```python
from build123d import *

# Parameters (mm, degrees)
BOSS_EXTRUDE1_DEPTH      = 4.5
BOSS_EXTRUDE1_DEPTH_BACK = 4.5
SKETCH3_R                = 1.75
CUT_EXTRUDE1_DEPTH       = 4
FILLET1_R                = 2
SKETCH4_R                = 8.25
CUT_EXTRUDE2_DEPTH       = 2.7
CUT_EXTRUDE2_DEPTH_BACK  = 2.7


with BuildPart() as part:
    # Sketch2 → Boss-Extrude1 (new body, two sides)
    with BuildSketch(Plane(origin=(0, 0, 0), x_dir=(0, 0, -1), z_dir=(1, 0, 0))) as boss_extrude1_sk:
        with BuildLine():
            Line((9.539392014, 1.5), (15.5, 1.5))
            Line((15.5, 1.5), (15.5, -1.5))
            Line((15.5, -1.5), (7, -1.5))
            ThreePointArc((7, -1.5), (0, 5.5), (-7, -1.5))
            Line((-7, -1.5), (-15.5, -1.5))
            Line((-15.5, -1.5), (-15.5, 1.5))
            Line((-15.5, 1.5), (-9.539392014, 1.5))
            ThreePointArc((-9.539392014, 1.5), (0, 8.5), (9.539392014, 1.5))
        make_face()
    extrude(amount=BOSS_EXTRUDE1_DEPTH)
    extrude(boss_extrude1_sk.sketch, amount=-BOSS_EXTRUDE1_DEPTH_BACK)

    # Sketch3 → Cut-Extrude1 (cut, through all)
    with BuildSketch(Plane(origin=(0, 1.5, 0), x_dir=(1, 0, 0), z_dir=(0, 1, 0))):
        with Locations((0, 12.5)):
            Circle(SKETCH3_R)
        with Locations((0, -12.5)):
            Circle(SKETCH3_R)
    extrude(amount=-CUT_EXTRUDE1_DEPTH, mode=Mode.SUBTRACT)

    # Fillet1
    fillet1_edges = [part.edges().sort_by_distance(p)[0] for p in [
        (4.5, 0, -15.5),
        (-4.5, 0, 15.5),
        (4.5, 0, 15.5),
        (-4.5, 0, -15.5),
    ]]
    fillet(fillet1_edges, radius=FILLET1_R)

    # Sketch4 → Cut-Extrude2 (cut, two sides)
    with BuildSketch(Plane(origin=(0, 0, 0), x_dir=(0, 0, -1), z_dir=(1, 0, 0))) as cut_extrude2_sk:
        with Locations((0, -1.5)):
            Circle(SKETCH4_R)
    extrude(amount=CUT_EXTRUDE2_DEPTH, mode=Mode.SUBTRACT)
    extrude(cut_extrude2_sk.sketch, amount=-CUT_EXTRUDE2_DEPTH_BACK, mode=Mode.SUBTRACT)


solid = part.part
```
The model under review builds one solid part; all positions refer to its coordinate system, in mm. A direction names the side the tool comes from. Round coordinates to 2 decimals unless told otherwise and drop trailing zeros. Loops run counter-clockwise (first coordinate to the right, second up) from the corner with the lowest first, then second, coordinate; pieces in that order, holes last. Notation, with made-up numbers: (-27.75, -36.5) -> (21.25, -36.5) arc R24 ccw to (21.25, -16.5) -> close; hole circle Ø3 at (20.25, -29). An arc over 180 degrees is marked (long way). Answer as a JSON object with one key per item and string values. Group by question number.
1) For line 1 (X direction, y = 0.6, z = -12.5); line 2 (Z direction, x = 0, y = -0.65); line 3 (X direction, y = 4, z = -5.5), list the stretches that pass through material, from the lowest coordinate up. Write a range as [from, to].
2) We need section B-B on z = 0. Write out the cut boundary in (x, y), then the cut area to 4 significant figures.
3) We need section D-D on y = 3.75. Write out the cut boundary in (x, z), then the cut area to 3 significant figures.
4) For pin 1 Ø1 at (y, z) = (6.5, -7) entering from -X; pin 2 Ø1.8 at (x, z) = (1.5, -12) entering from +Y, all flat-tipped, find the tip position at first contact; note any pin that passes through.
5) We need section C-C on y = 0. Write out the cut boundary in (x, z).
6) We need section A-A on z = -12.5. Write out the cut boundary in (x, y), then the cut area to 3 significant figures.
7) For faces 1 (the face through (3.93, -0.02, -14.9)), 2 (the face through (0.1, 1.5, 10.6)), 3 (the face through (0, 1.5, -10)), 4 (the face through (-3.93, -0.02, -14.9)), 5 (the face through (2.7, 6, 0)), list the 3-axis set-ups (+Z, -Z, +X, -X, +Y, -Y) from which the entire face can be reached by the end or side of a thin tool; tool diameter is ignored.
8) Mouldability with a two-part tool opening along Z and no side actions: class faces 6 (the face through (-2.7, 6, 0)), 7 (the face through (-4.5, 6, 0)), 8 (the face through (-3.93, 0.02, 14.9)), 9 (the face through (3.61, 5.5, -0.15)) as released by +Z, released by -Z, zero draft, split by the parting line, or undercut.
Result set:
{
 "1": {"line 1": "[-4.5, -1.75], [1.75, 4.5]", "line 2": "[-15.5, -14.25], [-10.75, -8.21], [8.21, 10.75], [14.25, 15.5]", "line 3": "[-4.5, -2.7], [2.7, 4.5]"},
 "2": {"outline": "(-4.5, 5.5) -> (-2.7, 5.5) -> (-2.7, 6.75) -> (2.7, 6.75) -> (2.7, 5.5) -> (4.5, 5.5) -> (4.5, 8.5) -> (-4.5, 8.5) -> close", "area": "20.25 mm²"},
 "3": {"outline": "(-4.5, -8.51) -> (4.5, -8.51) -> (4.5, -4.63) -> (2.7, -4.63) -> (2.7, -6.36) -> (-2.7, -6.36) -> (-2.7, -4.63) -> (-4.5, -4.63) -> close; (-4.5, 4.63) -> (-2.7, 4.63) -> (-2.7, 6.36) -> (2.7, 6.36) -> (2.7, 4.63) -> (4.5, 4.63) -> (4.5, 8.51) -> (-4.5, 8.51) -> close", "area": "51.1 mm²"},
 "4": {"pin 1": "through", "pin 2": "y = 1.5"},
 "5": {"outline": "(-4.5, -13.5) arc R2 ccw to (-2.5, -15.5) -> (2.5, -15.5) arc R2 ccw to (4.5, -13.5) -> (4.5, -6.84) -> (2.7, -6.84) -> (2.7, -8.11) -> (-2.7, -8.11) -> (-2.7, -6.84) -> (-4.5, -6.84) -> close; (-4.5, 6.84) -> (-2.7, 6.84) -> (-2.7, 8.11) -> (2.7, 8.11) -> (2.7, 6.84) -> (4.5, 6.84) -> (4.5, 13.5) arc R2 ccw to (2.5, 15.5) -> (-2.5, 15.5) arc R2 ccw to (-4.5, 13.5) -> close; hole circle Ø3.5 at (0, -12.5); hole circle Ø3.5 at (0, 12.5)"},
 "6": {"outline": "(-4.5, -1.5) -> (-1.75, -1.5) -> (-1.75, 1.5) -> (-4.5, 1.5) -> close; (1.75, -1.5) -> (4.5, -1.5) -> (4.5, 1.5) -> (1.75, 1.5) -> close", "area": "16.5 mm²"},
 "7": {"face 1": "-Z, +X, +Y, -Y", "face 2": "+Z, +X, -X, +Y", "face 3": "-Z, +X, -X, +Y", "face 4": "-Z, -X, +Y, -Y", "face 5": "-Y"},
 "8": {"face 6": "undercut", "face 7": "zero draft", "face 8": "released by +Z", "face 9": "undercut"}
}
